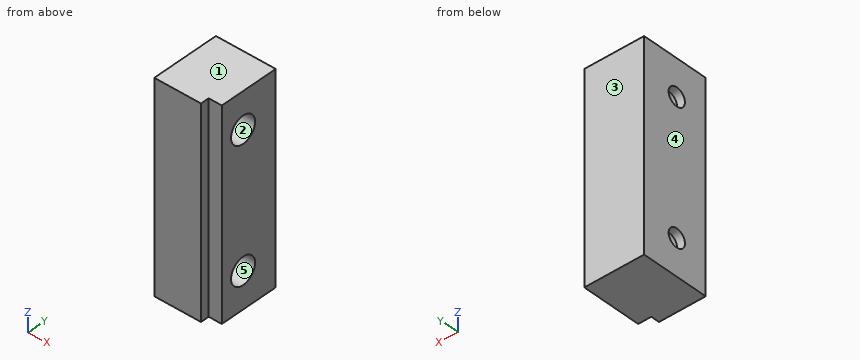
```python
from build123d import *

# Parameters (mm, degrees)
SKETCH1_W           = 44.45
SKETCH1_H           = 50.8
BOSS_EXTRUDE1_DEPTH = 76.2
CUT_EXTRUDE1_REACH  = 93.801
SKETCH2_R           = 6.731
SKETCH3_R           = 9.906
CUT_EXTRUDE2_DEPTH  = 38.608
SKETCH4_W           = 9.764994968
SKETCH4_H           = 6.35
CUT_EXTRUDE4_DEPTH  = 157.092506627


with BuildPart() as part:
    # Sketch1 → Boss-Extrude1 (new, symmetric)
    with BuildSketch(Plane.XY):
        Rectangle(SKETCH1_W, SKETCH1_H)
    extrude(amount=BOSS_EXTRUDE1_DEPTH, both=True)

    # Sketch2 → Cut-Extrude1 (cut, up to next)
    with BuildSketch(Plane(origin=(22.225, 0, 0), x_dir=(0, 0, -1), z_dir=(1, 0, 0)), mode=Mode.PRIVATE) as cut_extrude1_sk1:
        with Locations((-49.2125, -1.524)):
            Circle(SKETCH2_R)
    cut_extrude1_tool1 = extrude(cut_extrude1_sk1.sketch, amount=-CUT_EXTRUDE1_REACH, mode=Mode.PRIVATE) & part.part
    # Sketch2 → Cut-Extrude1 (cut, up to next)
    with BuildSketch(Plane(origin=(22.225, 0, 0), x_dir=(0, 0, -1), z_dir=(1, 0, 0)), mode=Mode.PRIVATE) as cut_extrude1_sk2:
        with Locations((49.2125, -1.524)):
            Circle(SKETCH2_R)
    cut_extrude1_tool2 = extrude(cut_extrude1_sk2.sketch, amount=-CUT_EXTRUDE1_REACH, mode=Mode.PRIVATE) & part.part
    add(cut_extrude1_tool1.solids().sort_by_distance((22.225, -1.524, 49.2125))[0], mode=Mode.SUBTRACT)
    add(cut_extrude1_tool2.solids().sort_by_distance((22.225, -1.524, -49.2125))[0], mode=Mode.SUBTRACT)

    # Sketch3 → Cut-Extrude2 (cut)
    with BuildSketch(Plane(origin=(22.225, 0, 0), x_dir=(0, 0, -1), z_dir=(1, 0, 0))):
        with Locations((-49.2125, -1.524)):
            Circle(SKETCH3_R)
        with Locations((49.2125, -1.524)):
            Circle(SKETCH3_R)
    extrude(amount=-CUT_EXTRUDE2_DEPTH, mode=Mode.SUBTRACT)

    # Sketch4 → Cut-Extrude4 (cut, through all)
    with BuildSketch(Plane.XY.offset(76.2)):
        with Locations((17.342502516, -22.225)):
            Rectangle(SKETCH4_W, SKETCH4_H)
    extrude(amount=-CUT_EXTRUDE4_DEPTH, mode=Mode.SUBTRACT)


solid = part.part
```
Here's how the part is built. I have some questions about the finished solid (model axes, mm). Face numbers are marked on the shaded views. A direction names the side the tool comes from. Give positions to 0.01 mm unless a question says otherwise; leave off trailing zeros. Order: outer loops, then holes, each group sorted by start corner. A loop starts at its lowest first (then second) coordinate and runs counter-clockwise, first axis right, second up. Notation, with made-up numbers: M 69,17.5 L 98,17.5 A25 ccw 98,38.5 Z; hole C -10,43 d10. An arc over 180 degrees is marked long. Use a Markdown table: item, result. Add a question column.
1. I need wall thicknesses on probe 1 along Z at (x, y) = (-20, -4); probe 2 along Z at (x, y) = (9, 1.5); probe 3 along X at (y, z) = (-9.5, -50.5) (3 decimals). Which ranges of each line are inside material? Lowest first, please. Write a range as from..to.
2. For pin 1 Ø5 at (x, z) = (15.5, 15) entering from -Y; pin 2 Ø10 at (y, z) = (-2, -46) entering from +X, each with a flat end and sliding along its axis, tell me the tip position at first contact or that it passes through.
3. Suppose I cut it at D-D (z = 0.5). List the corners of the cut face in (x, y) for me (3 decimals).
4. Suppose I cut it at A-A (z = -51.5). List the corners of the cut face in (x, y) for me (3 decimals).
5. On a 3-axis mill with a long thin cutter (end or side, diameter ignored), from which of +Z, -Z, +X, -X, +Y, -Y can I reach the whole of each face in a straight line? I mean the marked faces 1 and 2. Say none if no direction works.
6. Suppose I cut it at C-C (y = -21). List the corners of the cut face in (x, z) for me (3 decimals).
7. If we mould it in two halves opening along Y, with no side actions, what happens to the marked faces 3, 4 and 5? For each: +Y half, -Y half, draft (parallel to the pull), parting line (faces both ways), or undercut.
8. Suppose I cut it at B-B (x = 19). List the corners of the cut face in (y, z) for me, and give its area (3 significant figures).
Results list:
| question | item | result |
|---|---|---|
| 1 | probe 1 | z = -76.2..-55.47, -42.95..42.95, 55.47..76.2 |
| 1 | probe 2 | z = -76.2..-58.65, -39.78..39.78, 58.65..76.2 |
| 1 | probe 3 | x = -22.225..-16.383 |
| 2 | pin 1 | stops at y = -19.05 |
| 2 | pin 2 | stops at x = -16.38 |
| 3 | outline | M -22.225,-25.4 L 12.46,-25.4 L 12.46,-19.05 L 22.225,-19.05 L 22.225,25.4 L -22.225,25.4 Z |
| 4 | outline | M -22.225,-25.4 L 12.46,-25.4 L 12.46,-19.05 L 22.225,-19.05 L 22.225,-11.162 L -16.383,-11.162 L -16.383,-7.854 L -22.225,-7.854 Z; M -22.225,4.806 L -16.383,4.806 L -16.383,8.114 L 22.225,8.114 L 22.225,25.4 L -22.225,25.4 Z |
| 5 | face 1 | +Z, +X, -X, +Y, -Y |
| 5 | face 2 | +X |
| 6 | outline | M -22.225,-76.2 L 12.46,-76.2 L 12.46,76.2 L -22.225,76.2 Z |
| 7 | face 3 | +Y half |
| 7 | face 4 | draft |
| 7 | face 5 | undercut |
| 8 | outline | M -19.05,-76.2 L 25.4,-76.2 L 25.4,76.2 L -19.05,76.2 Z; hole C -1.52,-49.21 d19.81; hole C -1.52,49.21 d19.81 |
| 8 | area | 6,160 mm² |
